from build123d import *

# Parameters (mm, degrees)
SKETCH1_W          = 5
SKETCH1_H          = 150
BASE_FLANGE1_DEPTH = 50
EDGE_FLANGE2_DEPTH = 50
SKETCH2_W          = 40
SKETCH2_H          = 110
CUT_EXTRUDE1_DEPTH = 10
SKETCH6_R          = 1.75
CUT_EXTRUDE2_DEPTH = 10
SKETCH12_W         = 10
SKETCH12_H         = 30
CUT_EXTRUDE3_DEPTH = 10
CHAMFER1_SIZE      = 10
CHAMFER1_SIZE2     = 40
FILLET1_R          = 1
SKETCH17_W         = 80
SKETCH17_H         = 30
CUT_EXTRUDE6_DEPTH = 10
FILLET2_R          = 5


# Sheet-metal steps are written as plain solids
with BuildPart() as part:
    # Sketch1 → Base-Flange1 (new body)
    with BuildSketch(Plane.XY):
        with Locations((2.5, 75)):
            Rectangle(SKETCH1_W, SKETCH1_H)
    extrude(amount=BASE_FLANGE1_DEPTH)

    # Edge-Flange2 section (across the edge) → Edge-Flange2 (add)
    with BuildSketch(Plane(origin=(0, 168.652306326, 50), x_dir=(-0.6427876096865435, -0.7660444431189746, 0), z_dir=(0, 0, -1))):
        with BuildLine():
            Line((-5, 18.652306326), (-5, 157.668461709))
            Line((-5, 157.668461709), (0, 157.668461709))
            Line((0, 157.668461709), (0, 18.652306326))
            ThreePointArc((0, 18.652306326), (3.747688519, 1.747575857), (14.288495613, -11.989471399))
            Line((14.288495613, -11.989471399), (11.074557564, -15.819693614))
            ThreePointArc((11.074557564, -15.819693614), (-0.783850417, -0.365515452), (-5, 18.652306326))
        make_face()
    extrude(amount=EDGE_FLANGE2_DEPTH)

    # Sketch2 → Cut-Extrude1 (cut)
    with BuildSketch(Plane(origin=(5, 0, 0), x_dir=(0, 0, -1), z_dir=(1, 0, 0))):
        with Locations((-20, 55)):
            Rectangle(SKETCH2_W, SKETCH2_H)
    extrude(amount=-CUT_EXTRUDE1_DEPTH, mode=Mode.SUBTRACT)

    # Sketch6 → Cut-Extrude2 (cut)
    with BuildSketch(Plane.ZY):
        with Locations((30, 115)):
            Circle(SKETCH6_R)
        with Locations((5, 115)):
            Circle(SKETCH6_R)
        with Locations((5, 145)):
            Circle(SKETCH6_R)
        with Locations((30, 145)):
            Circle(SKETCH6_R)
    extrude(amount=-CUT_EXTRUDE2_DEPTH, mode=Mode.SUBTRACT)

    # Sketch12 → Cut-Extrude3 (cut)
    with BuildSketch(Plane.ZY):
        with Locations((45, 15)):
            Rectangle(SKETCH12_W, SKETCH12_H)
    extrude(amount=-CUT_EXTRUDE3_DEPTH, mode=Mode.SUBTRACT)

    # Chamfer1
    chamfer1_edges = [part.edges().sort_by_distance(p)[0] for p in [
        (-119.174079923, 271.914751059, 50),
    ]]
    chamfer1_side = [part.faces().sort_by_distance(p)[0] for p in [
        (-119.174079923, 271.914751059, 25),
    ]]
    chamfer(chamfer1_edges, length=CHAMFER1_SIZE, length2=CHAMFER1_SIZE2, reference=chamfer1_side[0])

    # Fillet1
    fillet1_edges = [part.edges().sort_by_distance(p)[0] for p in [
        (-88.532302198, 246.203246672, 50),
        (-119.174079923, 271.914751059, 40),
        (-119.174079923, 271.914751059, 0),
        (2.5, 110, 0),
        (2.5, 110, 40),
        (2.5, 30, 40),
        (2.5, 30, 50),
    ]]
    fillet(fillet1_edges, radius=FILLET1_R)

    # Sketch17 → Cut-Extrude6 (cut)
    with BuildSketch(Plane(origin=(86.258987465, 102.799458205, 0), x_dir=(0.7660444431189746, -0.6427876096865437, 0), z_dir=(0.6427876096865437, 0.7660444431189746, 0))):
        with Locations((-167.059919178, -27.5)):
            Rectangle(SKETCH17_W, SKETCH17_H)
    extrude(amount=-CUT_EXTRUDE6_DEPTH, mode=Mode.SUBTRACT)

    # Fillet2
    fillet2_edges = [part.edges().sort_by_distance(p)[0] for p in [
        (-12.681526588, 182.556888833, 12.5),
        (-12.681526588, 182.556888833, 42.5),
        (-73.965082038, 233.979897607, 42.5),
        (-73.965082038, 233.979897607, 12.5),
    ]]
    fillet(fillet2_edges, radius=FILLET2_R)


solid = part.part
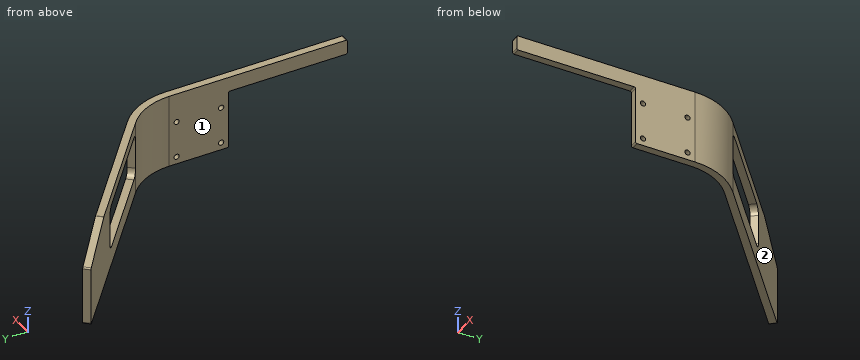
Verification items for the finished model (mm, model axes). Face numbers are marked on the shaded views. A direction names the side the tool comes from. Round coordinates to 2 decimals unless told otherwise and drop trailing zeros. Order: outer loops, then holes, each group sorted by start corner. A loop starts at its lowest first (then second) coordinate and runs counter-clockwise, first axis right, second up.
1. Thickness scan on L1, parallel to Z at x = 2.35, y = 115; L2, parallel to X at y = 113.5, z = 22; L3, parallel to X at y = 261, z = 28.5. Record the ranges inside material, lowest first.
Final values:
L1: z = 0 to 3.25, 6.75 to 28.25, 31.75 to 50
L2: x = 0 to 5
L3: x = -110.06 to -102.28
2. Section check D-D on x = -102.5. Record the cut outline in (y, z), then the cut area to 3 significant figures.
Final values:
outline: (254.66, 0) - (261.19, 0) - (261.19, 44.92) - (254.66, 45.97) - close
area: 297 mm2
3. Section check A-A on z = 10. Record the cut outline in (x, y).
Final values:
outline: (-120.78, 270) - (-14.29, 180.64) arc R40 cw to (0, 150) - (0, 110) - (5, 110) - (5, 150) arc R45 ccw to (-11.07, 184.47) - (-117.57, 273.83) - close
4. Go/stop test with flat-tipped pins: P1, Ø4, axis at y = 171.5, z = 40, coming from the +X side; P2, Ø8, axis at y = 141.5, z = 11.5, coming from the -X side; P3, Ø8, axis at x = -70, z = 33, coming from the +Y side; P4, Ø2, axis at y = 145, z = 5, coming from the +X side. Record where each tip stops, or that it passes through.
Final values:
P1: stops at x = 0.56
P2: stops at x = 0
P3: stops at y = 237.27
P4: passes through
5. Section check C-C on y = 168. Record the cut outline in (x, z).
Final values:
outline: (-4.28, 0) - (1.24, 0) - (1.24, 50) - (-4.28, 50) - close
6. Access from +Z, -Z, +X, -X, +Y, -Y to the whole of each face (thin tool, end or side, straight path). Record for the marked faces 1 and 2.
Final values:
face 1: +Z, -Z, -X, -Y
face 2: +Z, -Z, +X, +Y
7. Section check B-B on x = -22.5. Record the cut outline in (y, z).
Final values:
outline: (187.53, 0) - (194.06, 0) - (194.06, 12.5) - (187.53, 12.5) - close; (187.53, 42.5) - (194.06, 42.5) - (194.06, 50) - (187.53, 50) - close
